Could you check a few things on this model? Use its own coordinates, in mm. Face numbers are marked on the shaded views. A direction names the side the tool comes from. Give positions to 0.01 mm unless a question says otherwise; leave off trailing zeros. Loops run counter-clockwise (first coordinate to the right, second up) from the corner with the lowest first, then second, coordinate; pieces in that order, holes last. Notation, with made-up numbers: M 17.5,88.5 L 35.5,88.5 A22 cw 35.5,107.5 Z; hole C 86.5,-5 d11. An arc over 180 degrees is marked long. Answer in a Markdown table with one row per item. Add a question column.
1. Thinking about a two-plate mould opening in Z: for the marked faces 3, 4 and 5, which applies, released by +Z, released by -Z, zero draft, split by the parting line, or undercut?
2. Which directions (+Z, -Z, +X, -X, +Y, -Y) give clear straight access to the entire face, cutting with the end or side of a thin tool? Please do the marked faces 1 and 2.
3. I need wall thicknesses on line 1 along Z through (x, y) = (0.45, -2); line 2 along Y through (x, z) = (-1, 3); line 3 along X through (y, z) = (-0.4, 0.75). Which ranges of each line are inside material? Lowest first, please. Write a range as from..to.
4. If we section it at D-D on y = 2.05: List the corners of the cut face in (x, z) for me, then the cut area to 3 significant figures.
5. If we section it at C-C on z = 2.75: List the corners of the cut face in (x, y) for me, then the cut area to 3 significant figures.
6. If we section it at A-A on x = 0: List the corners of the cut face in (y, z) for me, then the cut area to 4 significant figures.
7. I'm going to push flat-ended pins straight in: pin 1 Ø3 at (x, z) = (1.5, 5) entering from +Y; pin 2 Ø1.5 at (x, z) = (0.5, 3.5) entering from +Y. Where does each tip first touch, or does it pass through?
```python
from build123d import *

# Parameters (mm, degrees)
F0_R     = 2.5
F1_DEPTH = 1
F2_R     = 1.7
F3_DEPTH = 5.5
F4_R     = 1.9
F5_DEPTH = 1
F6_SIZE  = 0.5


with BuildPart() as f1:
    # F0 (on Top) → F1 (new body)
    with BuildSketch(Plane.XY):
        Circle(F0_R)
    extrude(amount=F1_DEPTH)

    # F2 (on face) → F3 (join)
    with BuildSketch(Plane.XY.offset(1)):
        Circle(F2_R)
    extrude(amount=F3_DEPTH)

    # F4 (on face) → F5 (join)
    with BuildSketch(Plane.XY.offset(6.5)):
        Circle(F4_R)
    extrude(amount=-F5_DEPTH)

    # F6
    f6_edges = [f1.edges().sort_by_distance(p)[0] for p in [
        (-1.9, 0, 6.5),
    ]]
    chamfer(f6_edges, length=F6_SIZE)


solid = f1.part
```
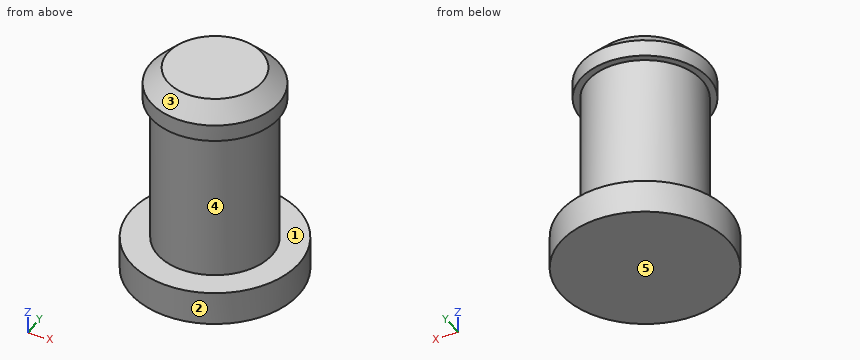
Results:
| question | item | result |
|---|---|---|
| 1 | face 3 | released by +Z |
| 1 | face 4 | undercut |
| 1 | face 5 | released by -Z |
| 2 | face 1 | none |
| 2 | face 2 | +Z, -Z |
| 3 | line 1 | 0..1 |
| 3 | line 2 | -1.37..1.37 |
| 3 | line 3 | -2.47..2.47 |
| 4 | outline | M -1.43,0 L 1.43,0 L 1.43,1 L -1.43,1 Z |
| 4 | area | 2.86 mm2 |
| 5 | outline | C 0,0 d3.4 |
| 5 | area | 9.08 mm2 |
| 6 | outline | M -2.5,0 L 2.5,0 L 2.5,1 L 1.7,1 L 1.7,5.5 L 1.9,5.5 L 1.9,6 L 1.4,6.5 L -1.4,6.5 L -1.9,6 L -1.9,5.5 L -1.7,5.5 L -1.7,1 L -2.5,1 Z |
| 6 | area | 23.85 mm2 |
| 7 | pin 1 | y = 1.9 |
| 7 | pin 2 | y = 1.7 |
